from build123d import *

# Parameters (mm, degrees)
SKETCH1_W                    = 104.775
SKETCH1_H                    = 53.63
BOSS_EXTRUDE1_DEPTH          = 6.35
F_0_257_DIAMETER_HOLE1_D     = 6.5278
FILLET1_R                    = 5
F_30_0_1285_DIAMETER_HOLE1_D = 3.2639


with BuildPart() as part:
    # Sketch1 → Boss-Extrude1 (new body)
    with BuildSketch(Plane(origin=(0, 0, 0), x_dir=(1, 0, 0), z_dir=(0, 1, 0))):
        with Locations((52.3875, 26.815)):
            Rectangle(SKETCH1_W, SKETCH1_H)
    extrude(amount=BOSS_EXTRUDE1_DEPTH)

    # F (0.257) Diameter Hole1 (through all)
    with Locations(Plane(origin=(0, 0, 0), x_dir=(-1, 0, 0), z_dir=(0, -1, 0))):
        with Locations((-52.385, 26.815)):
            Hole(F_0_257_DIAMETER_HOLE1_D / 2)

    # Fillet1
    fillet1_edges = [part.edges().sort_by_distance(p)[0] for p in [
        (0, 3.175, -53.63),
        (104.775, 3.175, -53.63),
        (104.775, 3.175, 0),
        (0, 3.175, 0),
    ]]
    fillet(fillet1_edges, radius=FILLET1_R)

    # #30 (0.1285) Diameter Hole1 (through all)
    with Locations(Plane(origin=(0, 0, 0), x_dir=(-1, 0, 0), z_dir=(0, -1, 0))):
        with Locations((-25.4, 6.1775), (-25.4, 47.4525), (-79.375, 47.4525), (-79.375, 6.1775)):
            Hole(F_30_0_1285_DIAMETER_HOLE1_D / 2)


solid = part.part
Part model, mm, in its own coordinate system. Coordinates: 2 decimals unless noted, no trailing zeros. Loops run counter-clockwise (first coordinate to the right, second up) from the corner with the lowest first, then second, coordinate; pieces in that order, holes last. Notation, with made-up numbers: M 22.5,62 L 40.5,62 A26 cw 40.5,99 Z; hole C 44.25,-10 d5. An arc over 180 degrees is marked long. Use a Markdown table: item, result. Add a question column.
Q1. Probe L1, parallel to Z at x = 25.4, y = 4.75; L2, parallel to X at y = 4.75, z = -46.5 (3 decimals); L3, parallel to X at y = 0.75, z = -26 (1 decimal). List the from-to ranges inside material, lowest first.
Q2. Mould opens along X. For faces 1 (the cylindrical face through (78.172, 3.219, -48.555)), 2 (the flat face through (0, 3, -27)), 3 (the cylindrical face through (103.271, 3.219, -52.204)), 4 (the flat face through (52, 3, 0)) say: +X half, -X half, draft (parallel to the pull), parting line (faces both ways), or undercut.
Q3. Cut at B-B (y = 4.75). Write the cut outline in (x, z) (1 decimal).
Q4. Cut at A-A (x = 25.4). Write the cut outline in (y, z), and give its area (3 significant figures).
Worked out:
| question | item | result |
|---|---|---|
| 1 | L1 | z = -53.63 to -49.08, -45.82 to -7.81, -4.55 to 0 |
| 1 | L2 | x = 0 to 24.075, 26.725 to 78.05, 80.7 to 104.775 |
| 1 | L3 | x = 0 to 49.2, 55.5 to 104.8 |
| 2 | face 1 | undercut |
| 2 | face 2 | -X half |
| 2 | face 3 | +X half |
| 2 | face 4 | draft |
| 3 | outline | M 0,-48.6 A5 ccw 5,-53.6 L 99.8,-53.6 A5 ccw 104.8,-48.6 L 104.8,-5 A5 ccw 99.8,0 L 5,0 A5 ccw 0,-5 Z; hole C 25.4,-47.5 d3.3; hole C 25.4,-6.2 d3.3; hole C 52.4,-26.8 d6.5; hole C 79.4,-47.5 d3.3; hole C 79.4,-6.2 d3.3 |
| 4 | outline | M 0,-53.63 L 6.35,-53.63 L 6.35,-49.08 L 0,-49.08 Z; M 0,-45.82 L 6.35,-45.82 L 6.35,-7.81 L 0,-7.81 Z; M 0,-4.55 L 6.35,-4.55 L 6.35,0 L 0,0 Z |
| 4 | area | 299 mm2 |
